Here's how the part is built. I have some questions about the finished solid (model axes, mm). A direction names the side the tool comes from. Give positions to 0.01 mm unless a question says otherwise; leave off trailing zeros. Loops run counter-clockwise (first coordinate to the right, second up) from the corner with the lowest first, then second, coordinate; pieces in that order, holes last.
Q1. For faces 1 (the face through (-386, 9, 0)), 2 (the face through (-687, 9, -88.9)), which set-ups out of +Z, -Z, +X, -X, +Y, -Y let a thin tool reach every point of the face, with its end or its side?
Q2. I need wall thicknesses on line 1 (Z direction, x = -640, y = 277.5); line 2 (X direction, y = 298, z = -213). Which ranges of each line are inside material? Lowest first, please.
Q3. Will these pins go through, and if not, where does the flat tip stop? P1, Ø4, axis at y = 199, z = -131.5, coming from the -X side; P2, Ø3, axis at y = 423.5, z = -162, coming from the +X side; P3, Ø12, axis at x = -652, y = -226.5, coming from the -Z side.
Q4. If we section it at A-A (y = 292): Please give me the cut outline in (x, z).
Q5. If we section it at B-B (z = -172): Please give me the cut outline in (x, y), plus the area to 3 significant figures.
from build123d import *

# Parameters (mm, degrees)
F0_W     = 762
F0_H     = 1244.6
F1_DEPTH = 228.6
F2_W     = 1244.6
F2_H     = 139.7
F3_DEPTH = 152.4


with BuildPart() as f1:
    # F0 (on Top) → F1 (new body)
    with BuildSketch(Plane.XY):
        with Locations((-381, 0)):
            Rectangle(F0_W, F0_H)
    extrude(amount=-F1_DEPTH)

    # F2 (on face) → F3 (cut)
    with BuildSketch(Plane(origin=(-762, 0, 0), x_dir=(0, -1, 0), z_dir=(-1, 0, 0))):
        with Locations((0, -158.75)):
            Rectangle(F2_W, F2_H)
    extrude(amount=-F3_DEPTH, mode=Mode.SUBTRACT)


solid = f1.part
Check sheet entries:
1. face 1: +Z, +X, -X, +Y, -Y
1. face 2: -Z, -X, +Y, -Y
2. line 1: z = -88.9 to 0
2. line 2: x = -609.6 to 0
3. P1: stops at x = -609.6
3. P2: stops at x = 0
3. P3: stops at z = -88.9
4. outline: (-762, -88.9) - (-609.6, -88.9) - (-609.6, -228.6) - (0, -228.6) - (0, 0) - (-762, 0) - close
5. outline: (-609.6, -622.3) - (0, -622.3) - (0, 622.3) - (-609.6, 622.3) - close
5. area: 759,000 mm2
